from build123d import *

# Parameters (mm, degrees)
EXTRUDE_1_DEPTH     = 3
CUT_EXTRUDE_1_REACH = 69.809
SKETCH_2_R          = 1.6
SKETCH_2_R_2        = 1.25
SKETCH_2_W          = 23
SKETCH_2_H          = 13
SKETCH_2_W_2        = 2
SKETCH_2_H_2        = 4
SKETCH_2_W_3        = 6
SKETCH_2_H_3        = 12


with BuildPart() as part:
    # 草图1 → 凸台-拉伸1 (new body)
    with BuildSketch(Plane(origin=(0, 0, 0), x_dir=(1, 0, 0), z_dir=(0, 1, 0))):
        Polygon((20, -20), (35, -20), (35, -38), (-35, -38), (-35, -20), (-20, -20), (-20, 20), (-20, 40), (-35, 40), (-35, 58), (35, 58), (35, 40), (20, 40), (20, 20), align=None)
    extrude(amount=EXTRUDE_1_DEPTH)

    # 草图2 → 切除-拉伸1 (cut, up to next)
    with BuildSketch(Plane(origin=(0, 3, 0), x_dir=(1, 0, 0), z_dir=(0, 1, 0)), mode=Mode.PRIVATE) as cut_extrude_1_sk1:
        with Locations(Location((-15.5, -15.5, 0), (0, 0, 270))):
            Circle(SKETCH_2_R)
    cut_extrude_1_tool1 = extrude(cut_extrude_1_sk1.sketch, amount=-CUT_EXTRUDE_1_REACH, mode=Mode.PRIVATE) & part.part
    # 草图2 → 切除-拉伸1 (cut, up to next)
    with BuildSketch(Plane(origin=(0, 3, 0), x_dir=(1, 0, 0), z_dir=(0, 1, 0)), mode=Mode.PRIVATE) as cut_extrude_1_sk2:
        with Locations(Location((-15.5, 15.5, 0), (0, 0, 270))):
            Circle(SKETCH_2_R)
    cut_extrude_1_tool2 = extrude(cut_extrude_1_sk2.sketch, amount=-CUT_EXTRUDE_1_REACH, mode=Mode.PRIVATE) & part.part
    # 草图2 → 切除-拉伸1 (cut, up to next)
    with BuildSketch(Plane(origin=(0, 3, 0), x_dir=(1, 0, 0), z_dir=(0, 1, 0)), mode=Mode.PRIVATE) as cut_extrude_1_sk3:
        with Locations(Location((15.5, -15.5, 0), (0, 0, 270))):
            Circle(SKETCH_2_R)
    cut_extrude_1_tool3 = extrude(cut_extrude_1_sk3.sketch, amount=-CUT_EXTRUDE_1_REACH, mode=Mode.PRIVATE) & part.part
    # 草图2 → 切除-拉伸1 (cut, up to next)
    with BuildSketch(Plane(origin=(0, 3, 0), x_dir=(1, 0, 0), z_dir=(0, 1, 0)), mode=Mode.PRIVATE) as cut_extrude_1_sk4:
        with Locations(Location((15.5, 15.5, 0), (0, 0, 270))):
            Circle(SKETCH_2_R)
    cut_extrude_1_tool4 = extrude(cut_extrude_1_sk4.sketch, amount=-CUT_EXTRUDE_1_REACH, mode=Mode.PRIVATE) & part.part
    # 草图2 → 切除-拉伸1 (cut, up to next)
    with BuildSketch(Plane(origin=(0, 3, 0), x_dir=(1, 0, 0), z_dir=(0, 1, 0)), mode=Mode.PRIVATE) as cut_extrude_1_sk5:
        with Locations(Location((-13.85, 26.5, 0), (0, 0, 270))):
            Circle(SKETCH_2_R_2)
    cut_extrude_1_tool5 = extrude(cut_extrude_1_sk5.sketch, amount=-CUT_EXTRUDE_1_REACH, mode=Mode.PRIVATE) & part.part
    # 草图2 → 切除-拉伸1 (cut, up to next)
    with BuildSketch(Plane(origin=(0, 3, 0), x_dir=(1, 0, 0), z_dir=(0, 1, 0)), mode=Mode.PRIVATE) as cut_extrude_1_sk6:
        with Locations(Location((13.85, 26.5, 0), (0, 0, 270))):
            Circle(SKETCH_2_R_2)
    cut_extrude_1_tool6 = extrude(cut_extrude_1_sk6.sketch, amount=-CUT_EXTRUDE_1_REACH, mode=Mode.PRIVATE) & part.part
    # 草图2 → 切除-拉伸1 (cut, up to next)
    with BuildSketch(Plane(origin=(0, 3, 0), x_dir=(1, 0, 0), z_dir=(0, 1, 0)), mode=Mode.PRIVATE) as cut_extrude_1_sk7:
        with Locations((0, 26.5)):
            Rectangle(SKETCH_2_W, SKETCH_2_H)
    cut_extrude_1_tool7 = extrude(cut_extrude_1_sk7.sketch, amount=-CUT_EXTRUDE_1_REACH, mode=Mode.PRIVATE) & part.part
    # 草图2 → 切除-拉伸1 (cut, up to next)
    with BuildSketch(Plane(origin=(0, 3, 0), x_dir=(1, 0, 0), z_dir=(0, 1, 0)), mode=Mode.PRIVATE) as cut_extrude_1_sk8:
        with Locations((-22, -33)):
            Rectangle(SKETCH_2_W_2, SKETCH_2_H_2)
    cut_extrude_1_tool8 = extrude(cut_extrude_1_sk8.sketch, amount=-CUT_EXTRUDE_1_REACH, mode=Mode.PRIVATE) & part.part
    # 草图2 → 切除-拉伸1 (cut, up to next)
    with BuildSketch(Plane(origin=(0, 3, 0), x_dir=(1, 0, 0), z_dir=(0, 1, 0)), mode=Mode.PRIVATE) as cut_extrude_1_sk9:
        with Locations((-29, -29)):
            Rectangle(SKETCH_2_W_3, SKETCH_2_H_3)
    cut_extrude_1_tool9 = extrude(cut_extrude_1_sk9.sketch, amount=-CUT_EXTRUDE_1_REACH, mode=Mode.PRIVATE) & part.part
    # 草图2 → 切除-拉伸1 (cut, up to next)
    with BuildSketch(Plane(origin=(0, 3, 0), x_dir=(1, 0, 0), z_dir=(0, 1, 0)), mode=Mode.PRIVATE) as cut_extrude_1_sk10:
        with Locations((-22, -25)):
            Rectangle(SKETCH_2_W_2, SKETCH_2_H_2)
    cut_extrude_1_tool10 = extrude(cut_extrude_1_sk10.sketch, amount=-CUT_EXTRUDE_1_REACH, mode=Mode.PRIVATE) & part.part
    # 草图2 → 切除-拉伸1 (cut, up to next)
    with BuildSketch(Plane(origin=(0, 3, 0), x_dir=(1, 0, 0), z_dir=(0, 1, 0)), mode=Mode.PRIVATE) as cut_extrude_1_sk11:
        with Locations((22, -33)):
            Rectangle(SKETCH_2_W_2, SKETCH_2_H_2)
    cut_extrude_1_tool11 = extrude(cut_extrude_1_sk11.sketch, amount=-CUT_EXTRUDE_1_REACH, mode=Mode.PRIVATE) & part.part
    # 草图2 → 切除-拉伸1 (cut, up to next)
    with BuildSketch(Plane(origin=(0, 3, 0), x_dir=(1, 0, 0), z_dir=(0, 1, 0)), mode=Mode.PRIVATE) as cut_extrude_1_sk12:
        with Locations((22, -25)):
            Rectangle(SKETCH_2_W_2, SKETCH_2_H_2)
    cut_extrude_1_tool12 = extrude(cut_extrude_1_sk12.sketch, amount=-CUT_EXTRUDE_1_REACH, mode=Mode.PRIVATE) & part.part
    # 草图2 → 切除-拉伸1 (cut, up to next)
    with BuildSketch(Plane(origin=(0, 3, 0), x_dir=(1, 0, 0), z_dir=(0, 1, 0)), mode=Mode.PRIVATE) as cut_extrude_1_sk13:
        with Locations((29, -29)):
            Rectangle(SKETCH_2_W_3, SKETCH_2_H_3)
    cut_extrude_1_tool13 = extrude(cut_extrude_1_sk13.sketch, amount=-CUT_EXTRUDE_1_REACH, mode=Mode.PRIVATE) & part.part
    # 草图2 → 切除-拉伸1 (cut, up to next)
    with BuildSketch(Plane(origin=(0, 3, 0), x_dir=(1, 0, 0), z_dir=(0, 1, 0)), mode=Mode.PRIVATE) as cut_extrude_1_sk14:
        with Locations((-22, 45)):
            Rectangle(SKETCH_2_W_2, SKETCH_2_H_2)
    cut_extrude_1_tool14 = extrude(cut_extrude_1_sk14.sketch, amount=-CUT_EXTRUDE_1_REACH, mode=Mode.PRIVATE) & part.part
    # 草图2 → 切除-拉伸1 (cut, up to next)
    with BuildSketch(Plane(origin=(0, 3, 0), x_dir=(1, 0, 0), z_dir=(0, 1, 0)), mode=Mode.PRIVATE) as cut_extrude_1_sk15:
        with Locations((-29, 49)):
            Rectangle(SKETCH_2_W_3, SKETCH_2_H_3)
    cut_extrude_1_tool15 = extrude(cut_extrude_1_sk15.sketch, amount=-CUT_EXTRUDE_1_REACH, mode=Mode.PRIVATE) & part.part
    # 草图2 → 切除-拉伸1 (cut, up to next)
    with BuildSketch(Plane(origin=(0, 3, 0), x_dir=(1, 0, 0), z_dir=(0, 1, 0)), mode=Mode.PRIVATE) as cut_extrude_1_sk16:
        with Locations((-22, 53)):
            Rectangle(SKETCH_2_W_2, SKETCH_2_H_2)
    cut_extrude_1_tool16 = extrude(cut_extrude_1_sk16.sketch, amount=-CUT_EXTRUDE_1_REACH, mode=Mode.PRIVATE) & part.part
    # 草图2 → 切除-拉伸1 (cut, up to next)
    with BuildSketch(Plane(origin=(0, 3, 0), x_dir=(1, 0, 0), z_dir=(0, 1, 0)), mode=Mode.PRIVATE) as cut_extrude_1_sk17:
        with Locations((22, 45)):
            Rectangle(SKETCH_2_W_2, SKETCH_2_H_2)
    cut_extrude_1_tool17 = extrude(cut_extrude_1_sk17.sketch, amount=-CUT_EXTRUDE_1_REACH, mode=Mode.PRIVATE) & part.part
    # 草图2 → 切除-拉伸1 (cut, up to next)
    with BuildSketch(Plane(origin=(0, 3, 0), x_dir=(1, 0, 0), z_dir=(0, 1, 0)), mode=Mode.PRIVATE) as cut_extrude_1_sk18:
        with Locations((22, 53)):
            Rectangle(SKETCH_2_W_2, SKETCH_2_H_2)
    cut_extrude_1_tool18 = extrude(cut_extrude_1_sk18.sketch, amount=-CUT_EXTRUDE_1_REACH, mode=Mode.PRIVATE) & part.part
    # 草图2 → 切除-拉伸1 (cut, up to next)
    with BuildSketch(Plane(origin=(0, 3, 0), x_dir=(1, 0, 0), z_dir=(0, 1, 0)), mode=Mode.PRIVATE) as cut_extrude_1_sk19:
        with Locations((29, 49)):
            Rectangle(SKETCH_2_W_3, SKETCH_2_H_3)
    cut_extrude_1_tool19 = extrude(cut_extrude_1_sk19.sketch, amount=-CUT_EXTRUDE_1_REACH, mode=Mode.PRIVATE) & part.part
    add(cut_extrude_1_tool1.solids().sort_by_distance((-15.5, 3, 15.5))[0], mode=Mode.SUBTRACT)
    add(cut_extrude_1_tool2.solids().sort_by_distance((-15.5, 3, -15.5))[0], mode=Mode.SUBTRACT)
    add(cut_extrude_1_tool3.solids().sort_by_distance((15.5, 3, 15.5))[0], mode=Mode.SUBTRACT)
    add(cut_extrude_1_tool4.solids().sort_by_distance((15.5, 3, -15.5))[0], mode=Mode.SUBTRACT)
    add(cut_extrude_1_tool5.solids().sort_by_distance((-13.85, 3, -26.5))[0], mode=Mode.SUBTRACT)
    add(cut_extrude_1_tool6.solids().sort_by_distance((13.85, 3, -26.5))[0], mode=Mode.SUBTRACT)
    add(cut_extrude_1_tool7.solids().sort_by_distance((0, 3, -26.5))[0], mode=Mode.SUBTRACT)
    add(cut_extrude_1_tool8.solids().sort_by_distance((-22, 3, 33))[0], mode=Mode.SUBTRACT)
    add(cut_extrude_1_tool9.solids().sort_by_distance((-29, 3, 29))[0], mode=Mode.SUBTRACT)
    add(cut_extrude_1_tool10.solids().sort_by_distance((-22, 3, 25))[0], mode=Mode.SUBTRACT)
    add(cut_extrude_1_tool11.solids().sort_by_distance((22, 3, 33))[0], mode=Mode.SUBTRACT)
    add(cut_extrude_1_tool12.solids().sort_by_distance((22, 3, 25))[0], mode=Mode.SUBTRACT)
    add(cut_extrude_1_tool13.solids().sort_by_distance((29, 3, 29))[0], mode=Mode.SUBTRACT)
    add(cut_extrude_1_tool14.solids().sort_by_distance((-22, 3, -45))[0], mode=Mode.SUBTRACT)
    add(cut_extrude_1_tool15.solids().sort_by_distance((-29, 3, -49))[0], mode=Mode.SUBTRACT)
    add(cut_extrude_1_tool16.solids().sort_by_distance((-22, 3, -53))[0], mode=Mode.SUBTRACT)
    add(cut_extrude_1_tool17.solids().sort_by_distance((22, 3, -45))[0], mode=Mode.SUBTRACT)
    add(cut_extrude_1_tool18.solids().sort_by_distance((22, 3, -53))[0], mode=Mode.SUBTRACT)
    add(cut_extrude_1_tool19.solids().sort_by_distance((29, 3, -49))[0], mode=Mode.SUBTRACT)


solid = part.part
Geometry: final body of the model. Coordinates: model frame, mm. A direction names the side the tool comes from. Coordinates: 2 decimals unless noted, no trailing zeros. Order: outer loops, then holes, each group sorted by start corner. A loop starts at its lowest first (then second) coordinate and runs counter-clockwise, first axis right, second up.
(1) Section query A-A (x = 27). Return the cut outline in (y, z), plus the area to 3 significant figures.
(2) Draft query along X for faces 1 (the face through (35, 1, 29)), 2 (the face through (-27, 1, -40)), 3 (the face through (-23, 2, -45)). Return one class per face: pulls with the +X half, pulls with the -X half, needs draft (parallel to the pull), parting line crosses it, or undercut.
(3) Section query D-D (x = 6). Return the cut outline in (y, z).
(4) Section query C-C (z = 15.5). Return the cut outline in (x, y), plus the area to 3 significant figures.
(5) Access query for faces 4 (the face through (21, 2, 25)), 5 (the face through (27, 1, 20)). Directions: +Z, -Z, +X, -X, +Y, -Y. A direction counts if a zero-diameter tool reaches every point of the face in a straight line with its end or side. Return the directions, or none.
(6) Material intervals for probe 1 along Z at (x, y) = (-31, 1.15); probe 2 along X at (y, z) = (2.2, 15.5); probe 3 along X at (y, z) = (1.65, -26.5), sorted ascending.
(7) Section query B-B (z = -26.5). Return the cut outline in (x, y), plus the area to 3 significant figures.
Solution:
1. outline: (0, -58) - (3, -58) - (3, -55) - (0, -55) - close; (0, -43) - (3, -43) - (3, -40) - (0, -40) - close; (0, 20) - (3, 20) - (3, 23) - (0, 23) - close; (0, 35) - (3, 35) - (3, 38) - (0, 38) - close
1. area: 36.0 mm2
2. face 1: pulls with the +X half
2. face 2: needs draft
2. face 3: undercut
3. outline: (0, -58) - (3, -58) - (3, -33) - (0, -33) - close; (0, -20) - (3, -20) - (3, 38) - (0, 38) - close
4. outline: (-20, 0) - (-17.1, 0) - (-17.1, 3) - (-20, 3) - close; (-13.9, 0) - (13.9, 0) - (13.9, 3) - (-13.9, 3) - close; (17.1, 0) - (20, 0) - (20, 3) - (17.1, 3) - close
4. area: 101 mm2
5. face 4: +Y, -Y
5. face 5: +X, +Y, -Y
6. probe 1: z = -58 to -55, -43 to -40, 20 to 23, 35 to 38
6. probe 2: x = -20 to -17.1, -13.9 to 13.9, 17.1 to 20
6. probe 3: x = -20 to -15.1, -12.6 to -11.5, 11.5 to 12.6, 15.1 to 20
7. outline: (-20, 0) - (-15.1, 0) - (-15.1, 3) - (-20, 3) - close; (-12.6, 0) - (-11.5, 0) - (-11.5, 3) - (-12.6, 3) - close; (11.5, 0) - (12.6, 0) - (12.6, 3) - (11.5, 3) - close; (15.1, 0) - (20, 0) - (20, 3) - (15.1, 3) - close
7. area: 36.0 mm2
